Autodesk Fusion 360 part; units mm, degrees
sketch "Sketch1" plane through (0, 0, 0) normal (0, 0, 1) x (1, 0, 0)
  line L0 (0, 0) -> (0, -609.6)
  line L1 (0, -609.6) -> (-304.8, -609.6)
  line L2 (-304.8, -609.6) -> (-304.8, -304.8)
  line L3 (-304.8, -304.8) -> (-609.6, -304.8)
  line L4 (-609.6, -304.8) -> (-609.6, 0)
  line L5 (-609.6, 0) -> (0, 0)
  line L6 (-403.5828, -304.8) -> (-304.8, -403.5828) construction
  line L7 (-354.1914, -354.1914) -> (0, 0) construction
  dimension "d1" = 609.6
  dimension "d2" = 609.6
  dimension "d3" = 304.8
  dimension "d4" = 304.8
  dimension "d17" = 135
  dimension "d18" = 139.7
extrude "Extrude1" add sketch "Sketch1" along normal blind 6.35
sketch "Sketch2" plane through (0, 0, 6.35) normal (0, 0, 1) x (-1, 0, 0)
  line L0 (609.6, 0) -> (609.6, 304.8)
  line L1 (609.6, 304.8) -> (304.8, 304.8)
  line L2 (304.8, 304.8) -> (304.8, 609.6)
  line L3 (304.8, 609.6) -> (0, 609.6)
  line L4 (0, 609.6) -> (0, 0)
  line L5 (0, 0) -> (609.6, 0)
  line L6 (304.8, 609.6) -> (254, 609.6)
  line L7 (254, 609.6) -> (254, 558.8)
  line L8 (254, 558.8) -> (304.8, 558.8)
  line L9 (304.8, 558.8) -> (304.8, 609.6)
  line L10 (0, 609.6) -> (50.8, 609.6)
  line L11 (50.8, 609.6) -> (50.8, 558.8)
  line L12 (50.8, 558.8) -> (0, 558.8)
  line L13 (0, 558.8) -> (0, 609.6)
  line L14 (0, 0) -> (50.8, 0)
  line L15 (50.8, 0) -> (50.8, 50.8)
  line L16 (50.8, 50.8) -> (0, 50.8)
  line L17 (0, 50.8) -> (0, 0)
  line L18 (609.6, 0) -> (558.8, 0)
  line L19 (558.8, 0) -> (558.8, 50.8)
  line L20 (558.8, 50.8) -> (609.6, 50.8)
  line L21 (609.6, 50.8) -> (609.6, 0)
  line L22 (609.6, 304.8) -> (558.8, 304.8)
  line L23 (558.8, 304.8) -> (558.8, 254)
  line L24 (558.8, 254) -> (609.6, 254)
  line L25 (609.6, 254) -> (609.6, 304.8)
  dimension "d7" = 50.8
  dimension "d8" = 50.8
  dimension "d9" = 50.8
  dimension "d10" = 50.8
  dimension "d11" = 50.8
  dimension "d12" = 50.8
extrude "Extrude2" add sketch "Sketch2" along normal blind 1981.2 contours L0 L5 L18 L19 L20 L21 | L0 L1 L22 L23 L24 L25 | L4 L5 L14 L15 L16 L17 | L3 L4 L10 L11 L12 L13 | L2 L3 L6 L7 L8 L9
sketch "Sketch3" plane through (0, 0, 1987.55) normal (0, 0, 1) x (-1, 0, 0)
  line L0 (0, 558.8) -> (50.8, 558.8)
  line L1 (50.8, 558.8) -> (50.8, 609.6)
  line L2 (50.8, 609.6) -> (0, 609.6)
  line L3 (0, 609.6) -> (0, 558.8)
  line L4 (0, 609.6) -> (0, 0)
  line L5 (0, 609.6) -> (304.8, 609.6)
  line L6 (304.8, 609.6) -> (304.8, 304.8)
  line L7 (304.8, 304.8) -> (609.6, 304.8)
  line L8 (609.6, 304.8) -> (609.6, 0)
  line L9 (609.6, 0) -> (0, 0)
  point P0 (304.8, 609.6)
  point P1 (609.6, 304.8)
extrude "Extrude3" add sketch "Sketch3" along normal blind 6.35
CAD build for the part. Positions are in the model's coordinates, mm. A direction names the side the tool comes from. Coordinates: 2 decimals unless noted, no trailing zeros. Loops run counter-clockwise (first coordinate to the right, second up) from the corner with the lowest first, then second, coordinate; pieces in that order, holes last. Notation, with made-up numbers: (-24.75, 27.5) - (30.25, 27.5) arc R29 cw to (30.25, 62.5) - close; hole circle Ø1 at (-35, 1.25). An arc over 180 degrees is marked (long way). Use CSV: the item, a comma, the result in double quotes. Start each with the question number.
Q1. 3-axis set-ups, long thin cutter, end or side, ignore diameter. For faces 4 (the flat face through (-241, -233, 6.35)), 5 (the flat face through (-584, -50.8, 983)), 6 (the flat face through (-558.8, -280, 983)): which of +Z, -Z, +X, -X, +Y, -Y reach the whole face in a straight line?
Q2. Probe probe 1 along Z at (x, y) = (-137, -116); probe 2 along X at (y, z) = (-579.5, 1854.5); probe 3 along X at (y, z) = (-29.5, 158.5). List the from-to ranges inside material, lowest first. Write a range as from..to.
Q3. Cut at B-B, the plane x = -91.5. List the corners of the cut face in (y, z), then the cut area to 3 significant figures.
Q4. Two-plate mould, pull along X, no slides. Class faces 1 (the flat face through (-279, -558.8, 983)), 2 (the flat face through (-50.8, -585, 983)), 3 (the flat face through (-609.6, -277, 992)): +X half, -X half, draft (parallel to the pull), parting line (faces both ways), or undercut.
Q5. Drop flat-ended pins along their axis: P1, Ø2, axis at x = -286, z = 971, coming from the +Y side; P2, Ø15, axis at y = -285, z = 743.5, coming from the +X side. Give the stop position or say it passes through.
Q6. Cut at A-A, the plane y = -347.5. List the corners of the cut face in (x, z), then the cut area to 3 significant figures.
Q7. Cut at C-C, the plane z = 1012. List the corners of the cut face in (x, y), then the cut area to 3 significant figures.
Here are the results:
1,face 4,"none"
1,face 5,"+X, -X"
1,face 6,"+X, +Y, -Y"
2,probe 1,"0..6.35, 1987.55..1993.9"
2,probe 2,"-304.8..-254, -50.8..0"
2,probe 3,"-609.6..-558.8, -50.8..0"
3,outline,"(-609.6, 0) - (0, 0) - (0, 6.35) - (-609.6, 6.35) - close; (-609.6, 1987.55) - (0, 1987.55) - (0, 1993.9) - (-609.6, 1993.9) - close"
3,area,"7,740 mm2"
4,face 1,"draft"
4,face 2,"undercut"
4,face 3,"-X half"
5,P1,"y = -558.8"
5,P2,"x = -558.8"
6,outline,"(-304.8, 0) - (0, 0) - (0, 6.35) - (-304.8, 6.35) - close; (-304.8, 1987.55) - (0, 1987.55) - (0, 1993.9) - (-304.8, 1993.9) - close"
6,area,"3,870 mm2"
7,outline,"(-609.6, -304.8) - (-558.8, -304.8) - (-558.8, -254) - (-609.6, -254) - close; (-609.6, -50.8) - (-558.8, -50.8) - (-558.8, 0) - (-609.6, 0) - close; (-304.8, -609.6) - (-254, -609.6) - (-254, -558.8) - (-304.8, -558.8) - close; (-50.8, -609.6) - (0, -609.6) - (0, -558.8) - (-50.8, -558.8) - close; (-50.8, -50.8) - (0, -50.8) - (0, 0) - (-50.8, 0) - close"
7,area,"12,900 mm2"
